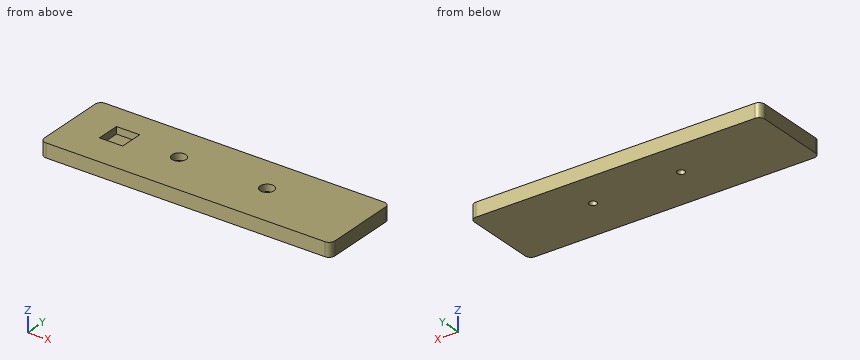
```python
from build123d import *

# Parameters (mm, degrees)
F0_W          = 250
F0_H          = 70
F1_DEPTH      = 12
F2_R          = 3.25
F3_DEPTH      = 25
F4_R          = 6
F5_DEPTH      = 6
F6_W          = 20
F6_H          = 20
F7_DEPTH      = 6
F8_W          = 20
F8_H          = 3
F9_DEPTH      = 20
F9_DEPTH_BACK = 25
F10_R         = 5


with BuildPart() as f1:
    # F0 (on Top) → F1 (new body)
    with BuildSketch(Plane.XY):
        with Locations((-3.651918, -3.040215)):
            Rectangle(F0_W, F0_H)
    extrude(amount=F1_DEPTH)

    # F2 (on face) → F3 (cut)
    with BuildSketch(Plane.XY.offset(12)):
        with Locations((-36.843423, 0)):
            Circle(F2_R)
        with Locations((38.979828, 0)):
            Circle(F2_R)
    extrude(amount=-F3_DEPTH, mode=Mode.SUBTRACT)

    # F4 (on face) → F5 (cut)
    with BuildSketch(Plane.XY.offset(12)):
        with Locations((-36.843423, 0)):
            Circle(F4_R)
        with Locations((38.979828, 0)):
            Circle(F4_R)
    extrude(amount=-F5_DEPTH, mode=Mode.SUBTRACT)

    # F6 (on face) → F7 (cut)
    with BuildSketch(Plane.XY.offset(12)):
        with Locations((-87.782149, -0.293668)):
            Rectangle(F6_W, F6_H)
    extrude(amount=-F7_DEPTH, mode=Mode.SUBTRACT)

    # F8 (on face) → F9 (cut, two sides)
    with BuildSketch(Plane(origin=(-77.782149, 0, 0), x_dir=(0, -1, 0), z_dir=(-1, 0, 0))) as f9_sk:
        with Locations((0.293668, 7.5)):
            Rectangle(F8_W, F8_H)
    extrude(amount=F9_DEPTH, mode=Mode.SUBTRACT)
    extrude(f9_sk.sketch, amount=-F9_DEPTH_BACK, mode=Mode.SUBTRACT)

    # F10
    f10_edges = [f1.edges().sort_by_distance(p)[0] for p in [
        (-128.651918, -38.040215, 6),
        (-128.651918, 31.959785, 6),
        (121.348082, -38.040215, 6),
        (121.348082, 31.959785, 6),
    ]]
    fillet(f10_edges, radius=F10_R)


solid = f1.part
```
Can you work these out from the model? Positions are in its coordinate system, mm. Coordinates: 2 decimals unless noted, no trailing zeros. Loops run counter-clockwise (first coordinate to the right, second up) from the corner with the lowest first, then second, coordinate; pieces in that order, holes last. Notation, with made-up numbers: M -29,-12 L -8,-12 A28 ccw -8,25 Z; hole C -20,16.25 d5. An arc over 180 degrees is marked long. Put each result on its own line as item: value. Start each with the question number.
(1) Will this pin go through, and if not, where does the flat tip stop? pin 1 Ø10.5 at (x, y) = (38.98, 0) entering from +Z.
(2) I need wall thicknesses on probe 1 along Z at (x, y) = (-66.5, -1.5); probe 2 along X at (y, z) = (-9.5, 10.75). Which ranges of each line are inside material? Lowest first, please.
(3) Imagine slicing it at A-A on y = 0. List the corners of the cut face in (x, z) for me, and give its area (3 significant figures).
Worked answers:
1. pin 1: stops at z = 6
2. probe 1: z = 0 to 6, 9 to 12
2. probe 2: x = -128.65 to -97.78, -77.78 to 121.35
3. outline: M -128.65,0 L -40.09,0 L -40.09,6 L -42.84,6 L -42.84,12 L -77.78,12 L -77.78,9 L -52.78,9 L -52.78,6 L -97.78,6 L -97.78,12 L -128.65,12 Z; M -33.59,0 L 35.73,0 L 35.73,6 L 32.98,6 L 32.98,12 L -30.84,12 L -30.84,6 L -33.59,6 Z; M 42.23,0 L 121.35,0 L 121.35,12 L 44.98,12 L 44.98,6 L 42.23,6 Z
3. area: 2,580 mm2
